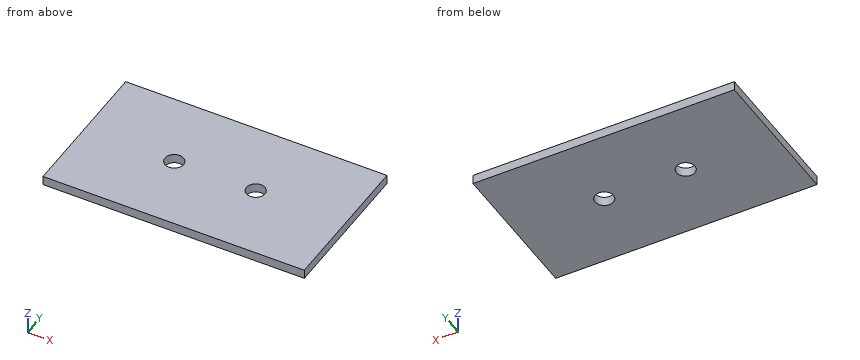
Autodesk Inventor part; units mm, degrees
ref_plane "YZ Plane" through (0, 0, 0) normal (1, 0, 0) x (0, 1, 0)
ref_plane "XZ Plane" through (0, 0, 0) normal (0, 1, 0) x (-1, 0, 0)
ref_plane "XY Plane" through (0, 0, 0) normal (0, 0, 1) x (1, 0, 0)
sketch "Sketch1" plane through (0, 0, 0) normal (0, 0, 1) x (1, 0, 0)
  line L0 (0, 0) -> (44.9013, 0)
  line L1 (44.9013, 0) -> (44.9013, 25.4)
  line L2 (44.9013, 25.4) -> (0, 25.4)
  line L3 (0, 25.4) -> (0, 0)
  line L4 (0, 12.7) -> (44.9013, 12.7) construction
  point P0 (15.4506, 12.7)
  point P1 (29.4506, 12.7)
  dimension "d0" = 44.9013
  dimension "d1" = 25.4
  dimension "d3" = 14
  dimension "d4" = 15.4506
  dimension "d5" = 15.4506
extrude "Plate1" add sketch "Sketch1" along normal blind 1.5875
hole "Hole1" at (15.4506, 12.7, 0) at (29.4506, 12.7, 0) direction (0, 0, 1) diameter 3.175 end through all
equation "\"d11\" = Thickness"
equation "\"BendRadius\" = Thickness"
equation "\"BendReliefWidth\" = Thickness"
equation "\"BendReliefDepth\" = 0.5 * Thickness"
equation "\"CornerReliefSize\" = 4 * Thickness"
equation "\"MinimumRemnant\" = 2 * Thickness"
equation "\"TransitionRadius\" = BendRadius"
equation "\"JacobiRadiusSize\" = BendRadius"
equation "\"GapSize\" = Thickness"
equation "\"d2\" = BendRadius"
properties part number "Bumper Rail Stand Top Cap"
Work out the finished part from the listing and answer in its coordinate system (mm). Give positions to 0.01 mm unless a question says otherwise; leave off trailing zeros. Write each loop counter-clockwise with the first axis right and the second up, starting at its lowest first coordinate (ties: lowest second). Pieces come first, ordered by that corner, then holes.
Q1. Given pin 1 (3 mm diameter, centred on x = 15.45, y = 12.7, fed in from +Z), flat-ended and moving along its own axis, determine where the tip first touches the part or whether it passes through.
Answer:
pin 1: passes through
Q2. The part is cut by section A-A on y = 12.7. Give the vertices of the cut face in (x, z), and give its area (3 significant figures).
Answer:
outline: (0, 0) - (13.86, 0) - (13.86, 1.59) - (0, 1.59) - close; (17.04, 0) - (27.86, 0) - (27.86, 1.59) - (17.04, 1.59) - close; (31.04, 0) - (44.9, 0) - (44.9, 1.59) - (31.04, 1.59) - close
area: 61.2 mm2
Q3. Straight lines are drawn through the part: L1, parallel to X at y = 12.7, z = 1.2; L2, parallel to Y at x = 29, z = 0.9; L3, parallel to Y at x = 16.5, z = 1. For each, find the intervals that lie inside material, in ascending order.
Answer:
L1: x = 0 to 13.86, 17.04 to 27.86, 31.04 to 44.9
L2: y = 0 to 11.18, 14.22 to 25.4
L3: y = 0 to 11.51, 13.89 to 25.4
